from build123d import *

# Parameters (mm, degrees)
SKETCH1_W        = 56.4
SKETCH1_H        = 56.4
EXTRUSION1_DEPTH = 76
THREAD4_D        = 5.5
THREAD4_DEPTH    = 8
THREAD4_TIP      = 1.652366702
SKETCH4_R        = 19.05
EXTRUSION2_DEPTH = 1.6
SKETCH5_R        = 3.175
EXTRUSION3_DEPTH = 21
SKETCH6_W        = 8
SKETCH6_H        = 8
EXTRUSION4_DEPTH = 71
FILLET1_R        = 2
FILLET2_R        = 2


with BuildPart() as part:
    # Sketch1 → Extrusion1 (new body)
    with BuildSketch(Plane.XY):
        Rectangle(SKETCH1_W, SKETCH1_H)
    extrude(amount=EXTRUSION1_DEPTH)

    # Thread4
    with Locations(Plane(origin=(0, 0, 0), x_dir=(-1, 0, 0), z_dir=(0, 0, -1))):
        with Locations((-23.57, 23.57), (23.57, 23.57), (23.57, -23.57), (-23.57, -23.57)):
            Hole(THREAD4_D / 2, depth=THREAD4_DEPTH)
            with Locations((0, 0, -(THREAD4_DEPTH + THREAD4_TIP / 2))):  # 118° drill point
                Cone(0, THREAD4_D / 2, THREAD4_TIP, mode=Mode.SUBTRACT)

    # Sketch4 → Extrusion2 (add)
    with BuildSketch(Plane(origin=(0, 0, 0), x_dir=(-1, 0, 0), z_dir=(0, 0, -1))):
        with Locations(Location((0, 0, 0), (0, 0, 180))):
            Circle(SKETCH4_R)
    extrude(amount=EXTRUSION2_DEPTH)

    # Sketch5 → Extrusion3 (add)
    with BuildSketch(Plane(origin=(0, 0, -1.6), x_dir=(-1, 0, 0), z_dir=(0, 0, -1))):
        with Locations(Location((0, 0, 0), (0, 0, 180))):
            Circle(SKETCH5_R)
    extrude(amount=EXTRUSION3_DEPTH)

    # Sketch6 → Extrusion4 (cut)
    with BuildSketch(Plane.XY.offset(76)):
        with Locations((-24.2, -24.2)):
            Rectangle(SKETCH6_W, SKETCH6_H)
        with Locations((24.2, -24.2)):
            Rectangle(SKETCH6_W, SKETCH6_H)
        with Locations((24.2, 24.2)):
            Rectangle(SKETCH6_W, SKETCH6_H)
        with Locations((-24.2, 24.2)):
            Rectangle(SKETCH6_W, SKETCH6_H)
    extrude(amount=-EXTRUSION4_DEPTH, mode=Mode.SUBTRACT)

    # Fillet1
    fillet1_edges = [part.edges().sort_by_distance(p)[0] for p in [
        (-28.2, 28.2, 2.5),
    ]]
    fillet(fillet1_edges, radius=FILLET1_R)

    # Fillet2
    fillet2_edges = [part.edges().sort_by_distance(p)[0] for p in [
        (-28.2, -28.2, 2.5),
        (-20.2, -20.2, 40.5),
        (-20.2, -28.2, 40.5),
        (-28.2, -20.2, 40.5),
        (28.2, -28.2, 2.5),
        (20.2, -20.2, 40.5),
        (28.2, -20.2, 40.5),
        (20.2, -28.2, 40.5),
        (28.2, 28.2, 2.5),
        (20.2, 20.2, 40.5),
        (20.2, 28.2, 40.5),
        (28.2, 20.2, 40.5),
        (-20.2, 20.2, 40.5),
        (-28.2, 20.2, 40.5),
        (-20.2, 28.2, 40.5),
    ]]
    fillet(fillet2_edges, radius=FILLET2_R)


solid = part.part
Check sheet for the modelled part. Datum: model origin and axes. Units: mm. A direction names the side the tool comes from. Give positions to 0.01 mm unless a question says otherwise; leave off trailing zeros. Write each loop counter-clockwise with the first axis right and the second up, starting at its lowest first coordinate (ties: lowest second). Pieces come first, ordered by that corner, then holes. Notation, with made-up numbers: (-30, -37) -> (14, -37) arc R12 ccw to (14, -23) -> close; hole circle Ø9 at (74.5, 86). An arc over 180 degrees is marked (long way). Write item = value, one per line.
Item 1: Sectioned sample at A-A on y = 23.57. Record the boundary of the cut face in (x, z), and give its area (3 significant figures).
Output:
outline = (-28.2, 0) -> (-26.32, 0) -> (-26.32, 5) -> (-28.2, 5) -> close; (-20.82, 0) -> (20.82, 0) -> (20.82, 5) -> (20.2, 5) -> (20.2, 76) -> (-20.2, 76) -> (-20.2, 5) -> (-20.82, 5) -> close; (26.32, 0) -> (28.2, 0) -> (28.2, 5) -> (26.32, 5) -> close
area = 3,100 mm^2
Item 2: Sectioned sample at D-D on y = 0. Record the boundary of the cut face in (x, z) (3 decimals), and give its area (3 significant figures).
Output:
outline = (-28.2, 0) -> (-19.05, 0) -> (-19.05, -1.6) -> (-3.175, -1.6) -> (-3.175, -22.6) -> (3.175, -22.6) -> (3.175, -1.6) -> (19.05, -1.6) -> (19.05, 0) -> (28.2, 0) -> (28.2, 76) -> (-28.2, 76) -> close
area = 4,480 mm^2
Item 3: Tool access check on faces 1 (the flat face through (20.2, 24, 41)), 2 (the cylindrical face through (-19.6, 27.63, 40)), 3 (the cylindrical face through (19.6, -27.63, 40)), 4 (the flat face through (-27, -24, 5)), 5 (the flat face through (-19.2, 0.4, 0)). Record the directions out of +Z, -Z, +X, -X, +Y, -Y that give a thin tool (end or side, any length) a straight path to the whole face; none if there is none.
Output:
face_1 = +Z, +X, +Y
face_2 = +Z, -X, +Y
face_3 = +Z, +X, -Y
face_4 = +Z, -X, -Y
face_5 = -Z
Item 4: Sectioned sample at B-B on z = 3. Record the boundary of the cut face in (x, y), and give its area (3 significant figures).
Output:
outline = (-28.2, -26.2) arc R2 ccw to (-26.2, -28.2) -> (26.2, -28.2) arc R2 ccw to (28.2, -26.2) -> (28.2, 26.2) arc R2 ccw to (26.2, 28.2) -> (-26.2, 28.2) arc R2 ccw to (-28.2, 26.2) -> close; hole circle Ø5.5 at (-23.57, -23.57); hole circle Ø5.5 at (-23.57, 23.57); hole circle Ø5.5 at (23.57, -23.57); hole circle Ø5.5 at (23.57, 23.57)
area = 3,080 mm^2
Item 5: Gauge pin test, flat ends, axial feed: pin 1 (3.5 mm diameter, centred on x = -23.57, y = -23.57, fed in from +Z); pin 2 (1 mm diameter, centred on x = 21.5, z = 50, fed in from +Y); pin 3 (6 mm diameter, centred on x = 15, y = -19.5, fed in from -Z); pin 4 (2 mm diameter, centred on x = -24.5, z = 29, fed in from -Y). Record the tip position at first contact, or that the pin passes through.
Output:
pin_1 = through
pin_2 = 20.6
pin_3 = 0
pin_4 = -20.2
Item 6: Scan lines: probe 1 along Y at (x, z) = (-23.57, 2.5); probe 2 along X at (y, z) = (23, 3); probe 3 along Z at (x, y) = (-18, 13). Record each from-to range of solid material in increasing order. Write a range as from..to.
Output:
probe_1 = -28.2..-26.32, -20.82..20.82, 26.32..28.2
probe_2 = -28.2..-26.26, -20.88..20.88, 26.26..28.2
probe_3 = 0..76
Item 7: Release check for a two-part mould opening along X. For faces 6 (the cylindrical face through (20.77, 20.8, 40)), 7 (the cylindrical face through (-20.8, -20.77, 40)), 8 (the flat face through (24, -20.2, 41)), 9 (the cylindrical face through (22.974, 20.885, 2.535)) record: +X half, -X half, draft (parallel to the pull), parting line (faces both ways), or undercut.
Output:
face_6 = +X half
face_7 = -X half
face_8 = draft
face_9 = undercut
